```python
from build123d import *

# Parameters (mm, degrees)
SKETCH1_W           = 76.3
SKETCH1_H           = 25.1
BOSS_EXTRUDE1_DEPTH = 2
SKETCH3_R           = 1
CUT_EXTRUDE2_DEPTH  = 10
SKETCH10_R          = 1.5
CUT_EXTRUDE8_DEPTH  = 2
CUT_EXTRUDE10_DEPTH = 0.4


with BuildPart() as part:
    # Sketch1 → Boss-Extrude1 (new body)
    with BuildSketch(Plane.XY):
        with Locations((38.15, 12.55)):
            Rectangle(SKETCH1_W, SKETCH1_H)
    extrude(amount=BOSS_EXTRUDE1_DEPTH)

    # Sketch3 → Cut-Extrude2 (cut)
    with BuildSketch(Plane.XY.offset(2)):
        with Locations((15, 21.1)):
            Circle(SKETCH3_R)
        with Locations((61.3, 4)):
            Circle(SKETCH3_R)
    extrude(amount=-CUT_EXTRUDE2_DEPTH, mode=Mode.SUBTRACT)

    # Sketch10 → Cut-Extrude8 (cut)
    with BuildSketch(Plane.XY.offset(2)):
        with Locations((20.5, 19.25108338)):
            Circle(SKETCH10_R)
        with Locations((20.5, 5.84891662)):
            Circle(SKETCH10_R)
        with Locations((54.5, 5.84891662)):
            Circle(SKETCH10_R)
        with Locations((54.5, 19.25108338)):
            Circle(SKETCH10_R)
        with Locations((33.5, 19.25108338)):
            Circle(SKETCH10_R)
        with Locations((41.5, 5.84891662)):
            Circle(SKETCH10_R)
        with Locations((34, 2.85)):
            Circle(SKETCH10_R)
        with Locations((34, 8.85)):
            Circle(SKETCH10_R)
        with Locations((41, 22.25)):
            Circle(SKETCH10_R)
        with Locations((41, 16.25)):
            Circle(SKETCH10_R)
    extrude(amount=-CUT_EXTRUDE8_DEPTH, mode=Mode.SUBTRACT)

    # Sketch12 → Cut-Extrude10 (cut)
    with BuildSketch(Plane.XY.offset(2)):
        Polygon((25.986752225, 19.834512657), (27.986752225, 19.834512657), (28.486752225, 19.545837522), (28.486752225, 18.923187791), (27.986752225, 18.634512657), (25.986752225, 18.634512657), (25.486752225, 18.923187791), (25.486752225, 19.545837522), align=None)
        Polygon((49.5, 6.15891662), (49.5, 5.53691662), (48.999437317, 5.24791662), (46.999437317, 5.24791662), (46.5, 5.537566351), (46.5, 6.159566351), (46.999437317, 6.44791662), (48.999437317, 6.44791662), align=None)
        Polygon((25.5, 6.159566351), (25.5, 5.537566351), (26.000562683, 5.248566351), (28.000562683, 5.248566351), (28.5, 5.537566351), (28.5, 6.160216081), (28.000562683, 6.448566351), (26.000562683, 6.448566351), align=None)
        Polygon((49.5, 19.56308338), (49.5, 18.94108338), (48.999437317, 18.65208338), (46.999437317, 18.65208338), (46.498874633, 18.94108338), (46.498874633, 19.56308338), (46.999437317, 19.85208338), (48.999437317, 19.85208338), align=None)
    extrude(amount=-CUT_EXTRUDE10_DEPTH, mode=Mode.SUBTRACT)


solid = part.part
```
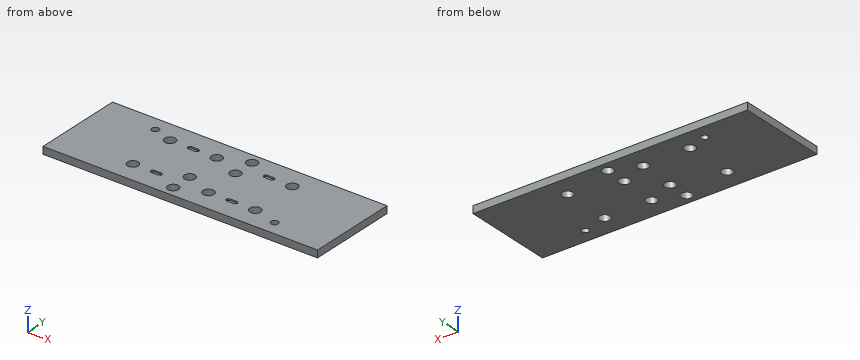
Source: CAD feature listing. Evaluate the final solid. Frame: model axes, mm. Give positions to 0.01 mm unless a question says otherwise; leave off trailing zeros. Write each loop counter-clockwise with the first axis right and the second up, starting at its lowest first coordinate (ties: lowest second). Pieces come first, ordered by that corner, then holes.
1. Section query D-D (x = 34). Return the cut outline in (y, z), then the cut area to 3 significant figures.
2. Section query A-A (y = 8.85). Return the cut outline in (x, z).
3. Section query B-B (x = 15). Return the cut outline in (y, z), then the cut area to 3 significant figures.
4. First-contact query: pin 1 (1.8 mm diameter, centred on x = 33.5, y = 19.25, fed in from +Z); pin 2 (0.6 mm diameter, centred on x = 48, y = 5.5, fed in from +Z). Flat tips, straight axial feed; report the tip coordinate or a pass-through.
5. Section query C-C (z = 0.5). Count the separate pieces of the cut face and the enclosed holes in it, then the cut area to 3 significant figures.
6. Material intervals for line 1 along X through (y, z) = (18.5, 0.6); line 2 along X through (y, z) = (21, 0.45); line 3 along Y through (x, z) = (61.3, 1.35), sorted ascending.
Output values:
1. outline: (0, 0) - (1.35, 0) - (1.35, 2) - (0, 2) - close; (4.35, 0) - (7.35, 0) - (7.35, 2) - (4.35, 2) - close; (10.35, 0) - (17.84, 0) - (17.84, 2) - (10.35, 2) - close; (20.67, 0) - (25.1, 0) - (25.1, 2) - (20.67, 2) - close
1. area: 32.5 mm2
2. outline: (0, 0) - (32.5, 0) - (32.5, 2) - (0, 2) - close; (35.5, 0) - (76.3, 0) - (76.3, 2) - (35.5, 2) - close
3. outline: (0, 0) - (20.1, 0) - (20.1, 2) - (0, 2) - close; (22.1, 0) - (25.1, 0) - (25.1, 2) - (22.1, 2) - close
3. area: 46.2 mm2
4. pin 1: passes through
4. pin 2: stops at z = 2
5. separate pieces: 1
5. enclosed holes: 12
5. area: 1,840 mm2
6. line 1: x = 0 to 19.2, 21.8 to 32.2, 34.8 to 53.2, 55.8 to 76.3
6. line 2: x = 0 to 14.01, 15.99 to 40.17, 41.83 to 76.3
6. line 3: y = 0 to 3, 5 to 25.1
